Geometry check sheet. Reference: the model listing, model coordinates, mm. A direction names the side the tool comes from. Coordinates: 2 decimals unless noted, no trailing zeros. Write each loop counter-clockwise with the first axis right and the second up, starting at its lowest first coordinate (ties: lowest second). Pieces come first, ordered by that corner, then holes.
Autodesk Inventor part; units mm, degrees
ref_plane "YZ Plane" through (0, 0, 0) normal (1, 0, 0) x (0, 1, 0)
ref_plane "XZ Plane" through (0, 0, 0) normal (0, 1, 0) x (-1, 0, 0)
ref_plane "XY Plane" through (0, 0, 0) normal (0, 0, 1) x (1, 0, 0)
sketch "Boceto1" plane through (0, 0, 0) normal (0, 0, 1) x (1, 0, 0)
  line L0 (0, 0) -> (130, 0)
  line L1 (130, 0) -> (130, -25)
  line L2 (130, -25) -> (0, -25)
  line L3 (0, -25) -> (0, 0)
  dimension "d0" = 130
  dimension "d1" = 25
extrude "Extrusión1" add sketch "Boceto1" along normal blind 5
sketch "Boceto2" plane through (0, 0, 5) normal (0, 0, 1) x (1, 0, 0)
  line L0 (130, 0) -> (130, -25)
  line L1 (0, -25) -> (0, 0)
  line L2 (-10, -7.5) -> (-10, -17.5)
  line L3 (140, -7.5) -> (140, -17.5)
  line L4 (0, -7.5) -> (0, -17.5)
  line L5 (130, -7.5) -> (130, -17.5)
  line L6 (140, -7.5) -> (130, -7.5)
  line L7 (0, -7.5) -> (-10, -7.5)
  line L8 (-10, -17.5) -> (0, -17.5)
  line L9 (130, -17.5) -> (140, -17.5)
  line L10 (0, 0) -> (130, 0)
  line L11 (130, -25) -> (0, -25)
  dimension "d5" = 10
  dimension "d6" = 10
  dimension "d12" = 7.5
  dimension "d13" = 10
  dimension "d14" = 10
  dimension "d15" = 7.5
extrude "Extrusión2" add sketch "Boceto2" against normal blind 5 contours L6 L3 L9 L0 | L1 L8 L2 L7
sketch "Boceto3" plane through (0, 0, 5) normal (0, 0, 1) x (1, 0, 0)
  circle A0 centre (65, -12.8431) radius 5
  line L0 (130, -17.5) -> (130, -25)
  dimension "d9" = 10
  dimension "d16" = 65
extrude "Extrusión3" cut sketch "Boceto3" against normal blind 5
properties part number "pieza lateral z refuerzo"
1. Gauge pin test, flat ends, axial feed: pin 1 Ø1.5 at (x, z) = (109.5, 2.5) entering from +Y; pin 2 Ø2.5 at (x, z) = (-4.5, 3.5) entering from -Y; pin 3 Ø2 at (y, z) = (-5.5, 0.5) entering from -X; pin 4 Ø9 at (x, y) = (65, -12.84) entering from -Z. Record the tip position at first contact, or that the pin passes through.
Computed values:
pin 1: stops at y = 0
pin 2: stops at y = -17.5
pin 3: stops at x = 0
pin 4: passes through
2. Thickness scan on line 1 along Y through (x, z) = (65, 2.4); line 2 along X through (y, z) = (-13, 2.6); line 3 along X through (y, z) = (-9, 2.1). Record the ranges inside material, lowest first.
Computed values:
line 1: y = -25 to -17.84, -7.84 to 0
line 2: x = -10 to 60, 70 to 140
line 3: x = -10 to 61.8, 68.2 to 140
3. Sectioned sample at A-A, the plane x = 65. Record the boundary of the cut face in (y, z), and give its area (3 significant figures).
Computed values:
outline: (-25, 0) - (-17.84, 0) - (-17.84, 5) - (-25, 5) - close; (-7.84, 0) - (0, 0) - (0, 5) - (-7.84, 5) - close
area: 75.0 mm2
4. Draft check along X on faces 1 (the flat face through (140, -12, 3)), 2 (the cylindrical face through (69.6, -14.8, 2.5)), 3 (the flat face through (0, -4, 2)). Enter one of: released by +X, released by -X, zero draft, split by the parting line, or undercut.
Computed values:
face 1: released by +X
face 2: undercut
face 3: released by -X
5. Sectioned sample at C-C, the plane z = 3.15. Record the boundary of the cut face in (x, y).
Computed values:
outline: (-10, -17.5) - (0, -17.5) - (0, -25) - (130, -25) - (130, -17.5) - (140, -17.5) - (140, -7.5) - (130, -7.5) - (130, 0) - (0, 0) - (0, -7.5) - (-10, -7.5) - close; hole circle Ø10 at (65, -12.84)
6. Sectioned sample at B-B, the plane y = -15.5. Record the boundary of the cut face in (x, z), and give its area (3 significant figures).
Computed values:
outline: (-10, 0) - (60.76, 0) - (60.76, 5) - (-10, 5) - close; (69.24, 0) - (140, 0) - (140, 5) - (69.24, 5) - close
area: 708 mm2
7. Access from +Z, -Z, +X, -X, +Y, -Y to the whole of each face (thin tool, end or side, straight path). Record for faces 4 (the flat face through (135, -7.5, 3)), 5 (the flat face through (130, -21, 2)), 6 (the flat face through (-5, -17.5, 3)), 7 (the flat face through (64, 0, 2)), 8 (the flat face through (-5, -7.5, 3)).
Computed values:
face 4: +Z, -Z, +X, +Y
face 5: +Z, -Z, +X, -Y
face 6: +Z, -Z, -X, -Y
face 7: +Z, -Z, +X, -X, +Y
face 8: +Z, -Z, -X, +Y
